from build123d import *

# Parameters (mm, degrees)
F0_W     = 4
F0_H     = 38.3
F0_R     = 1.75
F0_R_2   = 11.25
F1_DEPTH = 4
F3_DEPTH = 16
F4_R     = 2.75
F5_DEPTH = 4
F6_R     = 2.5
F7_W     = 0.5
F7_H     = 4
F8_DEPTH = 1


with BuildPart() as f1:
    # F0 (on Top) → F1 (new body)
    with BuildSketch(Plane.XY):
        with Locations((-23.15, 2)):
            Rectangle(F0_W, F0_H)
        Polygon((21.15, 21.15), (-21.15, 21.15), (-21.15, -17.15), (-21.15, -21.15), (21.15, -21.15), (21.15, -17.15), align=None)
        with Locations((-15.495, -15.495)):
            Circle(F0_R, mode=Mode.SUBTRACT)
        with Locations((15.495, -15.495)):
            Circle(F0_R, mode=Mode.SUBTRACT)
        with Locations((-15.495, 15.495)):
            Circle(F0_R, mode=Mode.SUBTRACT)
        Circle(F0_R_2, mode=Mode.SUBTRACT)
        with Locations((15.495, 15.495)):
            Circle(F0_R, mode=Mode.SUBTRACT)
        with Locations((23.15, 2)):
            Rectangle(F0_W, F0_H)
        Polygon((-21.15, -21.15), (-21.15, -17.15), (-25.15, -17.15), (-40.15, -17.15), (-40.15, -21.15), align=None)
        Polygon((25.15, -17.15), (21.15, -17.15), (21.15, -21.15), (40.15, -21.15), (40.15, -17.15), align=None)
    extrude(amount=F1_DEPTH)

    # F2 (on face) → F3 (join)
    with BuildSketch(Plane(origin=(0, 0, 0), x_dir=(1, 0, 0), z_dir=(0, 0, -1))):
        Polygon((-25.15, -21.15), (-21.15, -21.15), (-21.15, 17.15), (-21.15, 21.15), (-40.15, 21.15), (-40.15, 17.15), (-25.15, 17.15), align=None)
        Polygon((21.15, 17.15), (21.15, -21.15), (25.15, -21.15), (25.15, 17.15), (40.15, 17.15), (40.15, 21.15), (21.15, 21.15), align=None)
    extrude(amount=F3_DEPTH)

    # F4 (on face) → F5 (cut, through all)
    with BuildSketch(Plane.XZ.offset(21.15)):
        with Locations((-32.65, -6)):
            Circle(F4_R)
        with Locations((32.65, -6)):
            Circle(F4_R)
    extrude(amount=-F5_DEPTH, mode=Mode.SUBTRACT)

    # F6
    f6_edges = [f1.edges().sort_by_distance(p)[0] for p in [
        (-40.15, -19.15, 4),
        (-40.15, -19.15, -16),
        (40.15, -19.15, -16),
        (40.15, -19.15, 4),
        (25.15, -17.15, -6),
        (-25.15, -17.15, -6),
        (21.15, -21.15, -8),
        (-21.15, -21.15, -8),
    ]]
    fillet(f6_edges, radius=F6_R)

    # F7 (on face) → F8 (cut)
    with BuildSketch(Plane.XZ.offset(21.15)):
        with Locations((0.25, 2)):
            Rectangle(F7_W, F7_H)
        with Locations((-0.25, 2)):
            Rectangle(F7_W, F7_H)
    extrude(amount=-F8_DEPTH, mode=Mode.SUBTRACT)


solid = f1.part
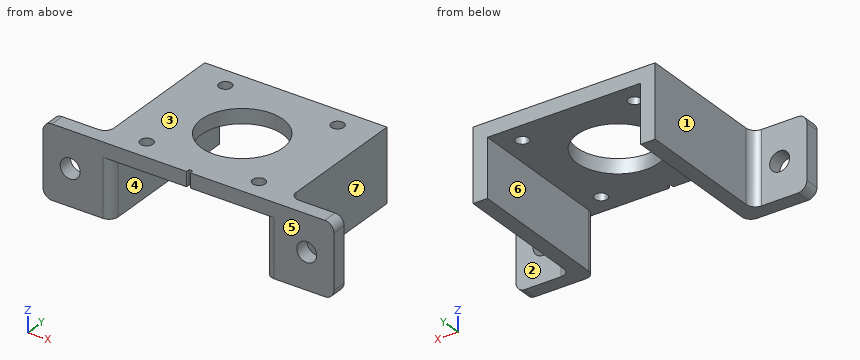
Here's how the part is built. I have some questions about the finished solid (model axes, mm). Face numbers are marked on the shaded views. A direction names the side the tool comes from. Coordinates: 2 decimals unless noted, no trailing zeros. Order: outer loops, then holes, each group sorted by start corner. A loop starts at its lowest first (then second) coordinate and runs counter-clockwise, first axis right, second up. Notation, with made-up numbers: M 34,83 L 92,83 A29 ccw 92,113 Z; hole C -10.75,2 d10. An arc over 180 degrees is marked long. Answer as CSV lines item,"result".
Item 1: For pin 1 (5 mm diameter, centred on x = -32.65, z = -6, fed in from +Y); pin 2 (4 mm diameter, centred on y = 10, z = -3.5, fed in from +X); pin 3 (6 mm diameter, centred on x = -33.5, z = -9, fed in from +Y); pin 4 (2 mm diameter, centred on y = -15, z = -8.5, fed in from -X), each with a flat end and sliding along its axis, tell me the tip position at first contact or that it passes through.
Results found:
pin 1,"through"
pin 2,"x = 25.15"
pin 3,"y = -17.15"
pin 4,"x = -25.55"
Item 2: We'd pull the mould along X, two halves only. Please class the marked faces 5, 6 and 7: +X half, -X half, draft (parallel to the pull), parting line (faces both ways), or undercut.
Results found:
face 5,"draft"
face 6,"undercut"
face 7,"+X half"
Item 3: If I drill on line 1 (Z direction, x = 32.65, y = -18.15); line 2 (X direction, y = 9, z = -1); line 3 (Y direction, x = -27.5, z = -5.25), over which ranges is the centre line in solid material (lowest first)?
Results found:
line 1,"-16 to -8.75, -3.25 to 4"
line 2,"-25.15 to -21.15, 21.15 to 25.15"
line 3,"-21.15 to -17.15"
Item 4: Imagine slicing it at C-C on y = 0. Write out the boundary of the cut face in (x, z).
Results found:
outline,"M -25.15,-16 L -21.15,-16 L -21.15,0 L -11.25,0 L -11.25,4 L -25.15,4 Z; M 11.25,0 L 21.15,0 L 21.15,-16 L 25.15,-16 L 25.15,4 L 11.25,4 Z"
Item 5: On a 3-axis mill with a long thin cutter (end or side, diameter ignored), from which of +Z, -Z, +X, -X, +Y, -Y can I reach the whole of each face in a straight line? I mean the marked faces 1, 2, 3 and 4. Say none if no direction works.
Results found:
face 1,"+Z, -Z, -X, +Y"
face 2,"+Z, -Z, +X, +Y"
face 3,"+Z, +X, -X, +Y, -Y"
face 4,"-Z, +Y, -Y"
Item 6: Imagine slicing it at B-B on z = -11.5. Write out the boundary of the cut face in (x, y), plus the area to 3 significant figures.
Results found:
outline,"M -40.15,-21.15 L -23.65,-21.15 A2.5 ccw -21.15,-18.65 L -21.15,21.15 L -25.15,21.15 L -25.15,-14.65 A2.5 cw -27.65,-17.15 L -40.15,-17.15 Z; M 21.15,-18.65 A2.5 ccw 23.65,-21.15 L 40.15,-21.15 L 40.15,-17.15 L 27.65,-17.15 A2.5 cw 25.15,-14.65 L 25.15,21.15 L 21.15,21.15 Z"
area,"458 mm2"
Item 7: Imagine slicing it at A-A on x = 32.65. Write out the boundary of the cut face in (y, z).
Results found:
outline,"M -21.15,-16 L -17.15,-16 L -17.15,-8.75 L -21.15,-8.75 Z; M -21.15,-3.25 L -17.15,-3.25 L -17.15,4 L -21.15,4 Z"
Item 8: Imagine slicing it at D-D on z = -6. Write out the boundary of the cut face in (x, y), plus the area to 3 significant figures.
Results found:
outline,"M -40.15,-21.15 L -35.4,-21.15 L -35.4,-17.15 L -40.15,-17.15 Z; M -29.9,-21.15 L -23.65,-21.15 A2.5 ccw -21.15,-18.65 L -21.15,21.15 L -25.15,21.15 L -25.15,-14.65 A2.5 cw -27.65,-17.15 L -29.9,-17.15 Z; M 21.15,-18.65 A2.5 ccw 23.65,-21.15 L 29.9,-21.15 L 29.9,-17.15 L 27.65,-17.15 A2.5 cw 25.15,-14.65 L 25.15,21.15 L 21.15,21.15 Z; M 35.4,-21.15 L 40.15,-21.15 L 40.15,-17.15 L 35.4,-17.15 Z"
area,"414 mm2"
